Source: CAD feature listing. Evaluate the final solid. Frame: model axes, mm. Give positions to 0.01 mm unless a question says otherwise; leave off trailing zeros. Write each loop counter-clockwise with the first axis right and the second up, starting at its lowest first coordinate (ties: lowest second). Pieces come first, ordered by that corner, then holes. Notation, with made-up numbers: (58.25, -13.5) -> (63.25, -13.5) arc R18 cw to (63.25, 13.5) -> close; hole circle Ø7 at (-2, 10.25). An arc over 180 degrees is marked (long way). Write item = value, one per line.
from build123d import *

# Parameters (mm, degrees)
F1_DEPTH       = 200
F3_D           = 5.5
F3_CSINK_D     = 11.2
F3_CSINK_ANGLE = 90


with BuildPart() as f1:
    # F0 (on Right) → F1 (new body)
    with BuildSketch(Plane.YZ):
        Polygon((1.8198511713, 5), (0, 0), (15, 0), (13.1801488287, 5), align=None)
    extrude(amount=F1_DEPTH)

    # F3 (through all)
    with Locations(Plane(origin=(0, 0, 0), x_dir=(1, 0, 0), z_dir=(0, 0, -1))):
        with Locations((30, -7.5), (170, -7.5)):
            CounterSinkHole(F3_D / 2, F3_CSINK_D / 2, counter_sink_angle=F3_CSINK_ANGLE)


solid = f1.part
(1) Section query A-A (y = 7.5). Return loops of the section in (x, z), plus the area to 3 significant figures.
Values follow:
outline = (0, 0) -> (24.4, 0) -> (27.25, 2.85) -> (27.25, 5) -> (0, 5) -> close; (32.75, 2.85) -> (35.6, 0) -> (164.4, 0) -> (167.25, 2.85) -> (167.25, 5) -> (32.75, 5) -> close; (172.75, 2.85) -> (175.6, 0) -> (200, 0) -> (200, 5) -> (172.75, 5) -> close
area = 929 mm2
(2) Pull-direction query (Y, two-part tool) for faces 1 (the face through (32.747, 7.379, 3.94)), 2 (the face through (200, 7, 3)), 3 (the face through (98.6, 14.1, 2.47)); classes: pulls with the +Y half, pulls with the -Y half, needs draft (parallel to the pull), parting line crosses it, or undercut.
Values follow:
face_1 = undercut
face_2 = needs draft
face_3 = pulls with the +Y half
(3) Section query C-C (z = 4.2). Return loops of the section in (x, y), plus the area to 3 significant figures.
Values follow:
outline = (0, 1.53) -> (200, 1.53) -> (200, 13.47) -> (0, 13.47) -> close; hole circle Ø5.5 at (30, 7.5); hole circle Ø5.5 at (170, 7.5)
area = 2,340 mm2
(4) Section query B-B (x = 30). Return loops of the section in (y, z).
Values follow:
outline = (0, 0) -> (1.9, 0) -> (4.75, 2.85) -> (4.75, 5) -> (1.82, 5) -> close; (10.25, 2.85) -> (13.1, 0) -> (15, 0) -> (13.18, 5) -> (10.25, 5) -> close
(5) Material intervals for line 1 (X direction, y = 5.5, z = 3.1); line 2 (X direction, y = 9, z = 1.7); line 3 (Y direction, x = 30, z = 3.6), sorted ascending.
Values follow:
line_1 = 0 to 28.11, 31.89 to 168.11, 171.89 to 200
line_2 = 0 to 26.4, 33.6 to 166.4, 173.6 to 200
line_3 = 1.31 to 4.75, 10.25 to 13.69
(6) First-contact query: pin 1 (1.5 mm diameter, centred on x = 114, z = 1.5, fed in from -Y); pin 2 (3 mm diameter, centred on x = 32.5, z = 3.5, fed in from +Y). Flat tips, straight axial feed; report the tip coordinate or a pass-through.
Values follow:
pin_1 = 0.27
pin_2 = 14.27
(7) Section query D-D (x = 77.5). Return loops of the section in (y, z), plus the area to 3 significant figures.
Values follow:
outline = (0, 0) -> (15, 0) -> (13.18, 5) -> (1.82, 5) -> close
area = 65.9 mm2
